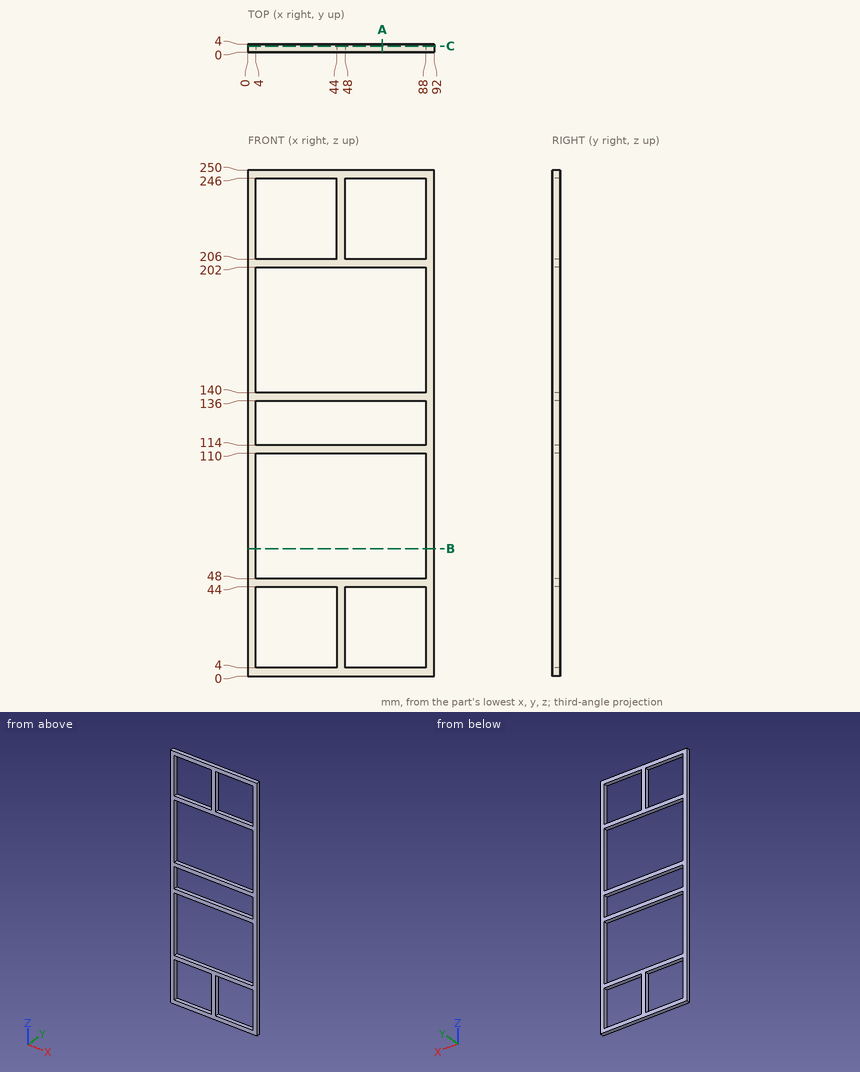
Part print with two shaded views. Sizes in mm from the minimum x, y, z corner. Round coordinates to 2 decimals unless told otherwise and drop trailing zeros. Order: outer loops, then holes, each group sorted by start corner. A loop starts at its lowest first (then second) coordinate and runs counter-clockwise, first axis right, second up.
(1) Drill centre lines: line 1 (X direction, y = 3.25, z = 231.5); line 2 (Z direction, x = 51, y = 3.85); line 3 (Z direction, x = 46.5, y = 2.2). Where is each one in solid material? Low to high.
(2) Band-saw the part on B-B (z = 63). List the corners of the cut face in (x, y), then the cut area to 3 significant figures.
(3) Band-saw the part on A-A (x = 66.5). List the corners of the cut face in (y, z), then the cut area to 3 significant figures.
(4) Band-saw the part on C-C (y = 3). Give the number of separate pieces and of enclosed holes in the cut face, then the cut area to 3 significant figures.
(5) Pin check, flat tip, straight feed: pin 1 (2 mm diameter, centred on y = 1.5, z = 121.5, fed in from -X). Stop position of the tip, or through.
Verdict:
1. line 1: x = 0 to 4, 44 to 48, 88 to 92
1. line 2: z = 0 to 4, 44 to 48, 110 to 114, 136 to 140, 202 to 206, 246 to 250
1. line 3: z = 0 to 48, 110 to 114, 136 to 140, 202 to 250
2. outline: (0, 0) - (4, 0) - (4, 4) - (0, 4) - close; (88, 0) - (92, 0) - (92, 4) - (88, 4) - close
2. area: 32.0 mm2
3. outline: (0, 0) - (4, 0) - (4, 4) - (0, 4) - close; (0, 44) - (4, 44) - (4, 48) - (0, 48) - close; (0, 110) - (4, 110) - (4, 114) - (0, 114) - close; (0, 136) - (4, 136) - (4, 140) - (0, 140) - close; (0, 202) - (4, 202) - (4, 206) - (0, 206) - close; (0, 246) - (4, 246) - (4, 250) - (0, 250) - close
3. area: 96.0 mm2
4. separate pieces: 1
4. enclosed holes: 7
4. area: 4,340 mm2
5. pin 1: stops at x = 0
